```python
from build123d import *

# Parameters (mm, degrees)
SKETCH1_W           = 140
SKETCH1_H           = 140
BOSS_EXTRUDE1_DEPTH = 3
SKETCH2_W           = 39.5
SKETCH2_H           = 3
SKETCH2_W_2         = 29
CUT_EXTRUDE2_DEPTH  = 3
SKETCH4_W           = 3
SKETCH4_H           = 16
CUT_EXTRUDE3_DEPTH  = 3
SKETCH6_R           = 1.47
CUT_EXTRUDE4_DEPTH  = 4
CUT_EXTRUDE5_DEPTH  = 3
SKETCH8_W           = 16
SKETCH8_H           = 3
CUT_EXTRUDE6_DEPTH  = 3
SKETCH9_R           = 5
BOSS_EXTRUDE3_DEPTH = 3
SKETCH10_R          = 2.12
CUT_EXTRUDE7_DEPTH  = 3


with BuildPart() as part:
    # Sketch1 → Boss-Extrude1 (new body)
    with BuildSketch(Plane(origin=(0, 0, 0), x_dir=(1, 0, 0), z_dir=(0, 1, 0))):
        Rectangle(SKETCH1_W, SKETCH1_H)
    extrude(amount=BOSS_EXTRUDE1_DEPTH)

    # Sketch2 → Cut-Extrude2 (cut)
    with BuildSketch(Plane(origin=(0, 3, 0), x_dir=(1, 0, 0), z_dir=(0, 1, 0))):
        with Locations((-50.25, 68.5)):
            Rectangle(SKETCH2_W, SKETCH2_H)
        with Locations((-50.25, -68.5)):
            Rectangle(SKETCH2_W, SKETCH2_H)
        with Locations((50.25, -68.5)):
            Rectangle(SKETCH2_W, SKETCH2_H)
        with Locations((50.25, 68.5)):
            Rectangle(SKETCH2_W, SKETCH2_H)
        with Locations((0, 68.5)):
            Rectangle(SKETCH2_W_2, SKETCH2_H)
        with Locations((0, -68.5)):
            Rectangle(SKETCH2_W_2, SKETCH2_H)
    extrude(amount=-CUT_EXTRUDE2_DEPTH, mode=Mode.SUBTRACT)

    # Sketch4 → Cut-Extrude3 (cut)
    with BuildSketch(Plane(origin=(0, 3, 0), x_dir=(1, 0, 0), z_dir=(0, 1, 0))):
        with Locations((-68.5, 22.5)):
            Rectangle(SKETCH4_W, SKETCH4_H)
        with Locations((-68.5, -22.5)):
            Rectangle(SKETCH4_W, SKETCH4_H)
        with Locations((68.5, 22.5)):
            Rectangle(SKETCH4_W, SKETCH4_H)
        with Locations((68.5, -22.5)):
            Rectangle(SKETCH4_W, SKETCH4_H)
    extrude(amount=-CUT_EXTRUDE3_DEPTH, mode=Mode.SUBTRACT)

    # Sketch6 → Cut-Extrude4 (cut, through all)
    with BuildSketch(Plane.XZ):
        with Locations((-22.5, 68.5)):
            Circle(SKETCH6_R)
        with Locations((22.5, 68.5)):
            Circle(SKETCH6_R)
    cut_extrude4 = extrude(amount=-CUT_EXTRUDE4_DEPTH, mode=Mode.SUBTRACT)

    # Mirror1: Cut-Extrude4 across plane
    add(cut_extrude4.mirror(Plane.XY), mode=Mode.SUBTRACT)

    # Sketch7 → Cut-Extrude5 (cut)
    with BuildSketch(Plane(origin=(0, 0, 0), x_dir=(-1, 0, 0), z_dir=(0, -1, 0))):
        Polygon((67, -23.97), (62.6, -23.97), (62.6, -25.75), (60, -25.75), (60, -23.97), (57.92, -23.97), (57.92, -21.03), (60, -21.03), (60, -19.25), (62.6, -19.25), (62.6, -21.03), (67, -21.03), align=None)
        Polygon((-67, -23.97), (-67, -21.03), (-62.6, -21.03), (-62.6, -19.25), (-60, -19.25), (-60, -21.03), (-57.92, -21.03), (-57.92, -23.97), (-60, -23.97), (-60, -25.75), (-62.6, -25.75), (-62.6, -23.97), align=None)
        Polygon((-67, 23.97), (-62.6, 23.97), (-62.6, 25.75), (-60, 25.75), (-60, 23.97), (-57.92, 23.97), (-57.92, 21.03), (-60, 21.03), (-60, 19.25), (-62.6, 19.25), (-62.6, 21.03), (-67, 21.03), align=None)
        Polygon((67, 23.97), (67, 21.03), (62.6, 21.03), (62.6, 19.25), (60, 19.25), (60, 21.03), (57.92, 21.03), (57.92, 23.97), (60, 23.97), (60, 25.75), (62.6, 25.75), (62.6, 23.97), align=None)
    extrude(amount=-CUT_EXTRUDE5_DEPTH, mode=Mode.SUBTRACT)

    # Sketch8 → Cut-Extrude6 (cut)
    with BuildSketch(Plane(origin=(0, 0, 0), x_dir=(-1, 0, 0), z_dir=(0, -1, 0))):
        with Locations((22.5, -68.5)):
            Rectangle(SKETCH8_W, SKETCH8_H)
    extrude(amount=-CUT_EXTRUDE6_DEPTH, mode=Mode.SUBTRACT)

    # Sketch9 → Boss-Extrude3 (add)
    with BuildSketch(Plane(origin=(0, 0, 0), x_dir=(-1, 0, 0), z_dir=(0, -1, 0))):
        with Locations((68.5, -68.5)):
            Circle(SKETCH9_R)
        with BuildLine():
            ThreePointArc((67.00186783, -67), (67.000933624, -67.000933624), (67, -67.00186783))
            Line((67, -67.00186783), (67, -67))
            Line((67, -67), (67.00186783, -67))
        make_face(mode=Mode.SUBTRACT)
        with BuildLine():
            ThreePointArc((67.00186783, -67), (68.5, -66.38), (69.99813217, -67))
            Line((69.99813217, -67), (67.00186783, -67))
        make_face(mode=Mode.SUBTRACT)
        with BuildLine():
            Line((69.99813217, -67), (70, -67))
            Line((70, -67), (70, -67.00186783))
            ThreePointArc((70, -67.00186783), (69.999066376, -67.000933624), (69.99813217, -67))
        make_face(mode=Mode.SUBTRACT)
    extrude(amount=-BOSS_EXTRUDE3_DEPTH)

    # Sketch10 → Cut-Extrude7 (cut)
    with BuildSketch(Plane(origin=(0, 3, 0), x_dir=(1, 0, 0), z_dir=(0, 1, 0))):
        with Locations((-68.5, -68.5)):
            Circle(SKETCH10_R)
    extrude(amount=-CUT_EXTRUDE7_DEPTH, mode=Mode.SUBTRACT)


solid = part.part
```
Check sheet for the modelled part. Datum: model origin and axes. Units: mm. Coordinates: 2 decimals unless noted, no trailing zeros. Order: outer loops, then holes, each group sorted by start corner. A loop starts at its lowest first (then second) coordinate and runs counter-clockwise, first axis right, second up. Notation, with made-up numbers: M -36,-16 L -21,-16 A23 cw -21,9 Z; hole C -31,-35.5 d7. An arc over 180 degrees is marked long. Write each question's results on one line, items separated by ' | '. Start each with the question number.
1. Cross-section at B-B on y = 0.5. State how many separate pieces and enclosed holes the cut face has, and give its area (3 significant figures).
2. Cross-section at C-C on z = 1.5. Record the cut outline in (x, y), and give its area (3 significant figures).
3. Mould release check, pull along Z, two halves, no side actions. Record for faces 1 (the face through (-1, 0, 1)), 2 (the face through (-68.57, 1.52, 70.62)): +Z half, -Z half, draft (parallel to the pull), parting line (faces both ways), or undercut.
4. Material ranges on probe 1 along Z at (x, y) = (-68.5, 1.85); probe 2 along X at (y, z) = (1.65, 68.5); probe 3 along Z at (x, y) = (-47, 0.25), recorded low to high.
5. Cross-section at A-A on x = -48.5. Record the cut outline in (y, z), and give its area (3 significant figures).
6. Go/stop test with flat-tipped pins: P1, Ø0.9, axis at y = 1.5, z = 20, coming from the +X side; P2, Ø1.3, axis at x = -61.5, y = 1.5, coming from the +Z side; P3, Ø1.5, axis at x = -38.5, y = 2.5, coming from the -Z side. Record where each tip stops, or that it passes through.
Checks:
1) separate pieces: 1 | enclosed holes: 4 | area: 18,600 mm²
2) outline: M -70,0 L 70,0 L 70,3 L -70,3 Z | area: 420 mm²
3) face 1: draft | face 2: undercut
4) probe 1: z = -67 to -30.5, -14.5 to 14.5, 30.5 to 66.38, 70.62 to 73.5 | probe 2: x = -73.5 to -70.62, -66.38 to -63.5, 14.5 to 21.03, 23.97 to 30.5 | probe 3: z = -67 to 67
5) outline: M 0,-67 L 3,-67 L 3,67 L 0,67 Z | area: 402 mm²
6) P1: stops at x = 67 | P2: stops at z = 67 | P3: stops at z = -67
